```python
from build123d import *

# Parameters (mm, degrees)
F1_W     = 25.4
F1_H     = 25.4
F2_DEPTH = 355.6
F3_T     = -1.5875
F4_DEPTH = 1.5885
F5_R     = 6.35
F6_DEPTH = 25.401


# Not quite as in the source:
# - a variable given as a bare number and used for a length is read in inches; the dataset says mm whatever the document's units were


with BuildPart() as f2:
    # F1 (on Top) → F2 (new body)
    with BuildSketch(Plane.XY):
        Rectangle(F1_W, F1_H)
    extrude(amount=F2_DEPTH)

    # F3
    f3_openings = [f2.faces().sort_by_distance(p)[0] for p in [
        (0, 0, 355.6),
    ]]
    offset(amount=F3_T, openings=f3_openings)

    # F4 (cut, through all): a face of the model
    f4_faces = [f2.faces().sort_by_distance(p)[0] for p in [
        (0, 0, 1.5875),
    ]]
    extrude(f4_faces, amount=-F4_DEPTH, mode=Mode.SUBTRACT)

    # F5 (on face) → F6 (cut, through all)
    with BuildSketch(Plane.XZ.offset(12.7)):
        with Locations((0, 152.4)):
            Circle(F5_R)
    extrude(amount=-F6_DEPTH, mode=Mode.SUBTRACT)


solid = f2.part
```
Verification items for the finished model (mm, model axes). A direction names the side the tool comes from. Give positions to 0.01 mm unless a question says otherwise; leave off trailing zeros. Order: outer loops, then holes, each group sorted by start corner. A loop starts at its lowest first (then second) coordinate and runs counter-clockwise, first axis right, second up. Notation, with made-up numbers: M 16.5,-4.5 L 39.5,-4.5 A26 cw 39.5,18.5 Z; hole C 64,27 d9. An arc over 180 degrees is marked long. Return JSON: item names as keys, results as strings. Group by question number.
1) Access from +Z, -Z, +X, -X, +Y, -Y to the whole of each face (thin tool, end or side, straight path). Record for faces 4 (the face through (-11.112, 0, 180)), 5 (the face through (12.7, 0, 175)).
2) Scan lines: line 1 (X direction, y = 1.75, z = 25.5); line 2 (Z direction, x = 0, y = -11.5). Record each from-to range of solid material in increasing order.
3) Section check C-C on z = 333. Record the cut outline in (x, y).
4) Section check B-B on y = 4. Record the cut outline in (x, z).
5) Section check D-D on x = 0. Record the cut outline in (y, z).
6) Mould release check, pull along Z, two halves, no side actions. Record for faces 1 (the face through (3.414, -11.917, 157.754)), 2 (the face through (0, -11.112, 180)), 3 (the face through (-11.3, 0.1, 0)): pulls with the +Z half, pulls with the -Z half, needs draft (parallel to the pull), parting line crosses it, or undercut.
7) Section check A-A on z = 152.4. Record the cut outline in (x, y).
Answer block:
{
 "1": {"face 4": "+Z, -Z", "face 5": "+Z, -Z, +X, +Y, -Y"},
 "2": {"line 1": "x = -12.7 to -11.11, 11.11 to 12.7", "line 2": "z = 0 to 146.05, 158.75 to 355.6"},
 "3": {"outline": "M -12.7,-12.7 L 12.7,-12.7 L 12.7,12.7 L -12.7,12.7 Z; hole M -11.11,-11.11 L 11.11,-11.11 L 11.11,11.11 L -11.11,11.11 Z"},
 "4": {"outline": "M -12.7,0 L -11.11,0 L -11.11,355.6 L -12.7,355.6 Z; M 11.11,0 L 12.7,0 L 12.7,355.6 L 11.11,355.6 Z"},
 "5": {"outline": "M -12.7,0 L -11.11,0 L -11.11,146.05 L -12.7,146.05 Z; M -12.7,158.75 L -11.11,158.75 L -11.11,355.6 L -12.7,355.6 Z; M 11.11,0 L 12.7,0 L 12.7,146.05 L 11.11,146.05 Z; M 11.11,158.75 L 12.7,158.75 L 12.7,355.6 L 11.11,355.6 Z"},
 "6": {"face 1": "undercut", "face 2": "needs draft", "face 3": "pulls with the -Z half"},
 "7": {"outline": "M -12.7,-12.7 L -6.35,-12.7 L -6.35,-11.11 L -11.11,-11.11 L -11.11,11.11 L -6.35,11.11 L -6.35,12.7 L -12.7,12.7 Z; M 6.35,-12.7 L 12.7,-12.7 L 12.7,12.7 L 6.35,12.7 L 6.35,11.11 L 11.11,11.11 L 11.11,-11.11 L 6.35,-11.11 Z"}
}
